Work out the finished part from the listing and answer in its coordinate system (mm). Face numbers are marked on the shaded views. A direction names the side the tool comes from. Coordinates: 2 decimals unless noted, no trailing zeros. Order: outer loops, then holes, each group sorted by start corner. A loop starts at its lowest first (then second) coordinate and runs counter-clockwise, first axis right, second up. Notation, with made-up numbers: (62.25, 30) - (113.25, 30) arc R31 ccw to (113.25, 64) - close; hole circle Ø7 at (28, -19). An arc over 180 degrees is marked (long way). Answer as a JSON object with one key per item and string values. Group by question number.
1) Find the intervals of material crossed by line 1 along X through (y, z) = (3.1, 0); line 2 along X through (y, z) = (8.6, 0); line 3 along Z through (x, y) = (2.5, 2.75), in increasing order.
2) Section A-A (x = 0) is taken. Count the separate pieces of the cut face and the enclosed holes in it, plus the area to 3 significant figures.
3) Each of these flat-tipped pins is pushed along its axis until it touches: P1, Ø5.5, axis at x = 0, z = -17.25, coming from the +Y side; P2, Ø4, axis at x = 18, y = 3.5, coming from the -Z side; P3, Ø4, axis at x = 17.25, z = 0, coming from the -Y side; P4, Ø2.5, axis at x = 0, z = -17.25, coming from the +Y side. Where does it stop, or does it pass through?
4) A tool of negligible diameter and unlimited length cuts with its end or side. For the marked faces 4, 5 and 6, from which of +Z, -Z, +X, -X, +Y, -Y can it reach the whole face along a straight path? Write none if from no direction.
5) The mould has two halves that part along X. Classify the marked faces 1, 2 and 3: released by +X, released by -X, zero draft, split by the parting line, or undercut.
6) Section B-B (y = 4.75) is taken. Give the vertices of the cut face in (x, z), plus the area to 3 significant figures.
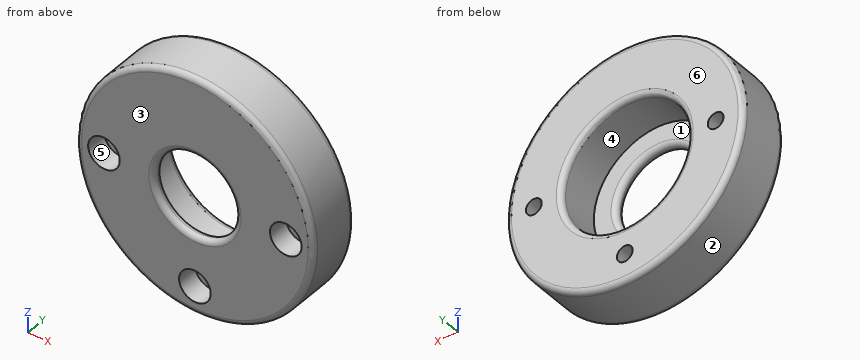
from build123d import *

# Parameters (mm, degrees)
SKETCH1_R           = 22.5
SKETCH1_R_2         = 1.5
BOSS_EXTRUDE1_DEPTH = 10
SKETCH2_R           = 12
CUT_EXTRUDE1_DEPTH  = 8
SKETCH3_R           = 7.75
CUT_EXTRUDE2_DEPTH  = 8
FILLET1_R           = 1
SKETCH4_R           = 3
CUT_EXTRUDE4_DEPTH  = 4


with BuildPart() as part:
    # Sketch1 → Boss-Extrude1 (new body)
    with BuildSketch(Plane(origin=(0, 0, 0), x_dir=(1, 0, 0), z_dir=(0, 1, 0))):
        with Locations(Location((0, 0, 0), (0, 0, 270))):
            Circle(SKETCH1_R)
        with Locations(Location((-17.25, 0, 0), (0, 0, 270))):
            Circle(SKETCH1_R_2, mode=Mode.SUBTRACT)
        with Locations(Location((0, 17.25, 0), (0, 0, 270))):
            Circle(SKETCH1_R_2, mode=Mode.SUBTRACT)
        with Locations(Location((17.25, 0, 0), (0, 0, 270))):
            Circle(SKETCH1_R_2, mode=Mode.SUBTRACT)
    extrude(amount=BOSS_EXTRUDE1_DEPTH)

    # Sketch2 → Cut-Extrude1 (cut)
    with BuildSketch(Plane(origin=(0, 10, 0), x_dir=(1, 0, 0), z_dir=(0, 1, 0))):
        with Locations(Location((0, 0, 0), (0, 0, 270))):
            Circle(SKETCH2_R)
    extrude(amount=-CUT_EXTRUDE1_DEPTH, mode=Mode.SUBTRACT)

    # Sketch3 → Cut-Extrude2 (cut)
    with BuildSketch(Plane(origin=(0, 2, 0), x_dir=(1, 0, 0), z_dir=(0, 1, 0))):
        with Locations(Location((0, 0, 0), (0, 0, 270))):
            Circle(SKETCH3_R)
    extrude(amount=-CUT_EXTRUDE2_DEPTH, mode=Mode.SUBTRACT)

    # Fillet1
    fillet1_edges = [part.edges().sort_by_distance(p)[0] for p in [
        (0, 10, -12),
        (0, 0, -7.75),
        (0, 2, -7.75),
        (0, 10, -22.5),
        (0, 0, -22.5),
    ]]
    fillet(fillet1_edges, radius=FILLET1_R - 0.0001)  # a hair under: the kernel refuses the full size

    # Sketch4 → Cut-Extrude4 (cut)
    with BuildSketch(Plane(origin=(0, 0, 0), x_dir=(1, 0, 0), z_dir=(0, 1, 0))):
        with Locations(Location((-17.25, 0, 0), (0, 0, 270))):
            Circle(SKETCH4_R)
        with Locations(Location((0, 17.25, 0), (0, 0, 270))):
            Circle(SKETCH4_R)
        with Locations(Location((17.25, 0, 0), (0, 0, 270))):
            Circle(SKETCH4_R)
    extrude(amount=CUT_EXTRUDE4_DEPTH, mode=Mode.SUBTRACT)


solid = part.part
Report:
{
 "1": {"line 1": "x = -22.5 to -20.25, -14.25 to -12, 12 to 14.25, 20.25 to 22.5", "line 2": "x = -22.5 to -18.75, -15.75 to -12, 12 to 15.75, 18.75 to 22.5", "line 3": "z = -22.36 to -18.91, -15.59 to -11.74, 11.74 to 22.36"},
 "2": {"separate pieces": "3", "enclosed holes": "0", "area": "183 mm²"},
 "3": {"P1": "stops at y = 10", "P2": "stops at z = -15.82", "P3": "stops at y = 4", "P4": "passes through"},
 "4": {"face 4": "+Y", "face 5": "-Y", "face 6": "+Z, -Z, +X, -X, +Y"},
 "5": {"face 1": "undercut", "face 2": "split by the parting line", "face 3": "zero draft"},
 "6": {"outline": "circle Ø45 at (0, 0); hole circle Ø3 at (-17.25, 0); hole circle Ø24 at (0, 0); hole circle Ø3 at (0, -17.25); hole circle Ø3 at (17.25, 0)", "area": "1,120 mm²"}
}
